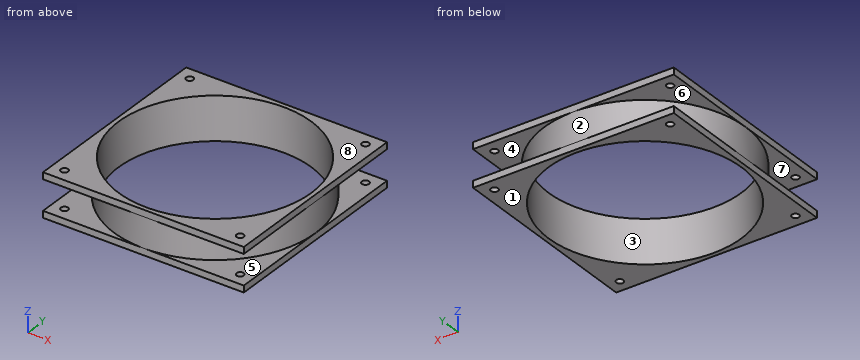
from build123d import *

# Parameters (mm, degrees)
F0_W     = 120
F0_H     = 120
F1_DEPTH = 26
F2_R     = 57.5
F3_DEPTH = 26.001
F6_DEPTH = 18
F7_R     = 2.15
F8_DEPTH = 26.001


with BuildPart() as f1:
    # F0 (on Top) → F1 (new body)
    with BuildSketch(Plane.XY):
        Rectangle(F0_W, F0_H)
    extrude(amount=F1_DEPTH)

    # F2 (on face) → F3 (cut, through all)
    with BuildSketch(Plane.XY.offset(26)):
        Circle(F2_R)
    extrude(amount=-F3_DEPTH, mode=Mode.SUBTRACT)

    # F5 (on offset) → F6 (cut)
    with BuildSketch(Plane.XY.offset(4)):
        with BuildLine():
            ThreePointArc((0, 60), (42.4264068712, 42.4264068712), (60, 0))
            Line((60, 0), (60, 60))
            Line((60, 60), (0, 60))
        make_face()
        with BuildLine():
            Line((60, -60), (60, 0))
            ThreePointArc((60, 0), (42.4264067803, -42.426406962), (-2.57e-07, -60))
            Line((-2.57e-07, -60), (60, -60))
        make_face()
        with BuildLine():
            Line((-60, -60), (-2.57e-07, -60))
            ThreePointArc((-2.57e-07, -60), (-42.4264070618, -42.4264066806), (-60, 2.822e-07))
            Line((-60, 2.822e-07), (-60, -60))
        make_face()
        with BuildLine():
            ThreePointArc((-60, 2.822e-07), (-42.4264067714, 42.426406971), (0, 60))
            Line((0, 60), (-60, 60))
            Line((-60, 60), (-60, 2.822e-07))
        make_face()
    extrude(amount=F6_DEPTH, mode=Mode.SUBTRACT)

    # F7 (on face) → F8 (cut, through all)
    with BuildSketch(Plane.XY.offset(26)):
        with Locations((-52.5, 52.5)):
            Circle(F7_R)
        with Locations((52.5, 52.5)):
            Circle(F7_R)
        with Locations((52.5, -52.5)):
            Circle(F7_R)
        with Locations((-52.5, -52.5)):
            Circle(F7_R)
    extrude(amount=-F8_DEPTH, mode=Mode.SUBTRACT)


solid = f1.part
Work out the finished part from the listing and answer in its coordinate system (mm). Face numbers are marked on the shaded views. A direction names the side the tool comes from. Coordinates: 2 decimals unless noted, no trailing zeros. Write each loop counter-clockwise with the first axis right and the second up, starting at its lowest first coordinate (ties: lowest second). Pieces come first, ordered by that corner, then holes. Notation, with made-up numbers: M 76,8 L 109,8 A8 ccw 109,14 Z; hole C 63,-23.5 d6. An arc over 180 degrees is marked long. Write item = value, one per line.
1. Flat-ended cylindrical pins translate along their axes: pin 1 (3.5 mm diameter, centred on x = 52.5, y = 52.5, fed in from +Z); pin 2 (8 mm diameter, centred on x = 18, z = 9, fed in from +Y); pin 3 (8 mm diameter, centred on x = 23.5, z = 10, fed in from -Y); pin 4 (10 mm diameter, centred on x = 30, z = 13, fed in from -Y). Find the tip coordinate at first contact, or state that the pin passes through.
Solution:
pin_1 = through
pin_2 = 58.34
pin_3 = -56.74
pin_4 = -54.54
2. The part is cut by section A-A (x = 26.5). Determine the outline of the cut face in (y, z), then the cut area to 3 significant figures.
Solution:
outline = M -60,0 L -51.03,0 L -51.03,26 L -60,26 L -60,22 L -53.83,22 L -53.83,4 L -60,4 Z; M 51.03,0 L 60,0 L 60,4 L 53.83,4 L 53.83,22 L 60,22 L 60,26 L 51.03,26 Z
area = 244 mm2
3. The part is cut by section D-D (z = 6.25). Determine the outline of the cut face in (x, y), then the cut area to 3 significant figures.
Solution:
outline = C 0,0 d120; hole C 0,0 d115
area = 923 mm2
4. The part is cut by section C-C (y = -52.5). State how many separate pieces and enclosed holes the cut face has, then the cut area to 3 significant figures.
Solution:
separate_pieces = 6
enclosed_holes = 0
area = 717 mm2
5. Determine the mould class of the marked faces 1, 2 and 3 for opening direction Y: released by +Y, released by -Y, zero draft, split by the parting line, or undercut.
Solution:
face_1 = zero draft
face_2 = split by the parting line
face_3 = undercut
6. For the marked faces 4, 5, 6, 7 and 8, determine the directions among +Z, -Z, +X, -X, +Y, -Y from which every point of the face is accessible in a straight line to the end or side of a thin tool.
Solution:
face_4 = +X, +Y
face_5 = +X, -Y
face_6 = -X, +Y
face_7 = -X, -Y
face_8 = +Z, +X, -X, +Y, -Y
7. Straight lines are drawn through the part: line 1 (Z direction, x = -38.5, y = -51.5); line 2 (Y direction, x = -52.5, z = 22.9); line 3 (Y direction, x = 0, z = 5). For each, find the intervals that lie inside material, in ascending order. Write a range as from..to.
Solution:
line_1 = 0..4, 22..26
line_2 = -60..-54.65, -50.35..-23.45, 23.45..50.35, 54.65..60
line_3 = -60..-57.5, 57.5..60
8. The part is cut by section B-B (y = -24.5). Determine the outline of the cut face in (x, z), then the cut area to 3 significant figures.
Solution:
outline = M -60,0 L -52.02,0 L -52.02,26 L -60,26 L -60,22 L -54.77,22 L -54.77,4 L -60,4 Z; M 52.02,0 L 60,0 L 60,4 L 54.77,4 L 54.77,22 L 60,22 L 60,26 L 52.02,26 Z
area = 227 mm2
